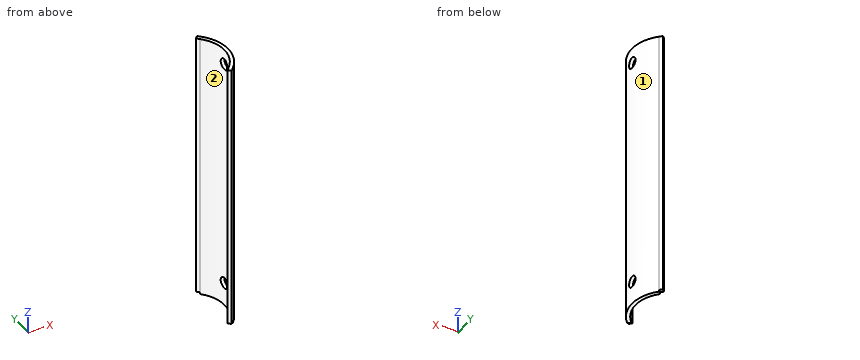
```python
from build123d import *

# Parameters (mm, degrees)
EXTRUDE1_DEPTH     = 74
SKETCH8_R          = 1.5
CUT_EXTRUDE4_DEPTH = 76.079920085
SKETCH9_W          = 74
SKETCH9_H          = 1
EXTRUDE2_DEPTH     = 1
SKETCH10_W         = 1
SKETCH10_H         = 74
EXTRUDE3_DEPTH     = 1
SKETCH12_W         = 0.495242112
SKETCH12_H         = 1
CUT_EXTRUDE5_DEPTH = 1
SKETCH13_W         = 1
SKETCH13_H         = 0.498210359
CUT_EXTRUDE6_DEPTH = 1


with BuildPart() as part:
    # Sketch1 → Extrude1 (new body)
    with BuildSketch(Plane.XY):
        with BuildLine():
            Line((6.618519472, 6.618519472), (7.325626253, 7.325626253))
            ThreePointArc((7.325626253, 7.325626253), (10.36, 0), (7.325626253, -7.325626253))
            Line((7.325626253, -7.325626253), (6.618519472, -6.618519472))
            ThreePointArc((6.618519472, -6.618519472), (9.36, 0), (6.618519472, 6.618519472))
        make_face()
    extrude(amount=EXTRUDE1_DEPTH)

    # Sketch8 → Cut-Extrude4 (cut, through all)
    with BuildSketch(Plane(origin=(0, 0, 0), x_dir=(0, 0, -1), z_dir=(1, 0, 0))):
        with Locations(Location((-6.35, 0, 0), (0, 0, 180))):
            Circle(SKETCH8_R)
        with Locations(Location((-69.85, 0, 0), (0, 0, 180))):
            Circle(SKETCH8_R)
    extrude(amount=CUT_EXTRUDE4_DEPTH, mode=Mode.SUBTRACT)

    # Sketch9 → Extrude2 (add)
    with BuildSketch(Plane(origin=(0, 0, 0), x_dir=(0, 0, 1), z_dir=(-0.7071067811865479, 0.7071067811865472, 0))):
        with Locations((37, 9.86)):
            Rectangle(SKETCH9_W, SKETCH9_H)
    extrude(amount=EXTRUDE2_DEPTH)

    # Sketch10 → Extrude3 (add)
    with BuildSketch(Plane(origin=(0, 0, 0), x_dir=(0.7071067811865475, -0.7071067811865477, 0), z_dir=(-0.7071067811865477, -0.7071067811865475, 0))):
        with Locations((9.86, 37)):
            Rectangle(SKETCH10_W, SKETCH10_H)
    extrude(amount=EXTRUDE3_DEPTH)

    # Sketch12 → Cut-Extrude5 (cut)
    with BuildSketch(Plane(origin=(-0.7071067811865468, 0.7071067811865459, 0), x_dir=(0, 0, 1), z_dir=(-0.7071067811865479, 0.7071067811865472, 0))):
        with Locations((0.247621056, 9.86)):
            Rectangle(SKETCH12_W, SKETCH12_H)
    extrude(amount=-CUT_EXTRUDE5_DEPTH, mode=Mode.SUBTRACT)

    # Sketch13 → Cut-Extrude6 (cut)
    with BuildSketch(Plane(origin=(6.618519472, -6.618519472, 0), x_dir=(-0.7071067811865476, -0.7071067811865476, 0), z_dir=(-0.7071067811865476, 0.7071067811865476, 0))):
        with Locations((0.5, 0.24910518)):
            Rectangle(SKETCH13_W, SKETCH13_H)
    extrude(amount=-CUT_EXTRUDE6_DEPTH, mode=Mode.SUBTRACT)


solid = part.part
```
Read the model definition and answer for the solid it produces. Units are mm, in the model's axes. Face numbers are marked on the shaded views. Coordinates: 2 decimals unless noted, no trailing zeros. Loops run counter-clockwise (first coordinate to the right, second up) from the corner with the lowest first, then second, coordinate; pieces in that order, holes last.
(1) The mould has two halves that part along Y. Classify the marked faces 1 and 2: released by +Y, released by -Y, zero draft, split by the parting line, or undercut.
Solution:
face 1: split by the parting line
face 2: undercut
(2) The part is cut by section D-D (z = 38.5). Determine the outline of the cut face in (x, y).
Solution:
outline: (5.91, -7.33) - (6.62, -8.03) - (7.33, -7.33) arc R10.36 ccw to (7.33, 7.33) - (6.62, 8.03) - (5.91, 7.33) - (6.62, 6.62) arc R9.36 cw to (6.62, -6.62) - close
(3) Consider line 1 along Y through (x, z) = (9.5, 69.85); line 2 along Y through (x, z) = (8.55, 41.5); line 3 along X through (y, z) = (-4.75, 65). Determine where each line is inside the solid, lowest interval first.
Solution:
line 1: y = -4.13 to -1.5, 1.5 to 4.13
line 2: y = -5.85 to -3.81, 3.81 to 5.85
line 3: x = 8.07 to 9.21
(4) The part is cut by section C-C (x = 8.2). Determine the outline of the cut face in (y, z), and give its area (3 significant figures).
Solution:
outline: (-6.33, 0) - (-4.51, 0) - (-4.51, 74) - (-6.33, 74) - close; (4.51, 0) - (6.33, 0) - (6.33, 74) - (4.51, 74) - close
area: 269 mm2
(5) The part is cut by section B-B (z = 69.85). Determine the outline of the cut face in (x, y).
Solution:
outline: (5.91, -7.33) - (6.62, -8.03) - (7.33, -7.33) arc R10.36 ccw to (10.25, -1.5) - (9.24, -1.5) arc R9.36 cw to (6.62, -6.62) - close; (5.91, 7.33) - (6.62, 6.62) arc R9.36 cw to (9.24, 1.5) - (10.25, 1.5) arc R10.36 ccw to (7.33, 7.33) - (6.62, 8.03) - close
(6) The part is cut by section A-A (y = 0). Determine the outline of the cut face in (x, z).
Solution:
outline: (9.36, 0) - (10.36, 0) - (10.36, 4.85) - (9.36, 4.85) - close; (9.36, 7.85) - (10.36, 7.85) - (10.36, 68.35) - (9.36, 68.35) - close; (9.36, 71.35) - (10.36, 71.35) - (10.36, 74) - (9.36, 74) - close
(7) Flat-ended cylindrical pins translate along their axes: pin 1 Ø1.6 at (x, y) = (6.5, 7.5) entering from -Z; pin 2 Ø2 at (x, z) = (8, 64) entering from +Y; pin 3 Ø8 at (y, z) = (1, 7.5) entering from -X; pin 4 Ø2 at (y, z) = (-2, 53.5) entering from -X. Find the tip coordinate at first contact, or state that the pin passes through.
Solution:
pin 1: stops at z = 0
pin 2: stops at y = 7.65
pin 3: stops at x = 7.91
pin 4: stops at x = 8.87
